from build123d import *

# Parameters (mm, degrees)
SKETCH004_R       = 3.1
PAD001_DEPTH      = 1
PAD001_DEPTH_BACK = 4
SKETCH_R          = 4.1
SKETCH_R_2        = 4
SKETCH_R_3        = 2
PAD_DEPTH         = 12
POCKET_DEPTH      = 70.501
SKETCH002_R       = 3.2
POCKET001_DEPTH   = 1


with BuildPart() as pad001:
    # Sketch004 → Pad001 (new body, two sides)
    with BuildSketch(Plane.XY.offset(5)) as pad001_sk:
        with Locations((0, -29.5)):
            Circle(SKETCH004_R)
    extrude(amount=PAD001_DEPTH)
    extrude(pad001_sk.sketch, amount=-PAD001_DEPTH_BACK)


with BuildPart() as cut:
    # Sketch → Pad (new body)
    with BuildSketch(Plane.XY):
        Polygon((-35.25, 35.05), (-35.25, 19.05), (-5, -35.45), (5, -35.45), (35.25, 19.05), (35.25, 35.05), (23.25, 35.05), (23.25, 23.05), (6, 23.05), (6, 35.05), (-6, 35.05), (-6, 23.05), (-23.25, 23.05), (-23.25, 35.05), align=None)
        with Locations((-29.25, 29.05)):
            Circle(SKETCH_R, mode=Mode.SUBTRACT)
        with Locations((0, 29.05)):
            Circle(SKETCH_R_2, mode=Mode.SUBTRACT)
        with Locations((29.25, 29.05)):
            Circle(SKETCH_R, mode=Mode.SUBTRACT)
        with Locations((-29.25, 19.05)):
            Circle(SKETCH_R_3, mode=Mode.SUBTRACT)
        with Locations((29.25, 19.05)):
            Circle(SKETCH_R_3, mode=Mode.SUBTRACT)
        with Locations((0, -29.45)):
            Circle(SKETCH_R_3, mode=Mode.SUBTRACT)
    extrude(amount=PAD_DEPTH)

    # Sketch001 → Pocket (cut, through all)
    with BuildSketch(Plane(origin=(-35.25, 0, 0), x_dir=(0, -1, 0), z_dir=(-1, 0, 0))):
        Polygon((-19.05, 12), (44.95, 0), (44.95, 12), align=None)
    extrude(amount=-POCKET_DEPTH, mode=Mode.SUBTRACT)

    # Sketch002 → Pocket001 (cut)
    with BuildSketch(Plane.XY.offset(12)):
        with Locations((-29.25, 19.05)):
            Circle(SKETCH002_R)
        with Locations((29.25, 19.05)):
            Circle(SKETCH002_R)
    extrude(amount=-POCKET001_DEPTH, mode=Mode.SUBTRACT)

    # Cut: cut Pad001
    add(pad001.part, mode=Mode.SUBTRACT)


solid = cut.part
Verification items for the finished model (mm, model axes). A direction names the side the tool comes from. Round coordinates to 2 decimals unless told otherwise and drop trailing zeros. Order: outer loops, then holes, each group sorted by start corner. A loop starts at its lowest first (then second) coordinate and runs counter-clockwise, first axis right, second up.
1. Release check for a two-part mould opening along Y. For faces 1 (the flat face through (31, 21, 11)), 2 (the flat face through (15, 23.05, 6)), 3 (the flat face through (-23.25, 29, 6)), 4 (the flat face through (0, -35.45, 1)) record: +Y half, -Y half, draft (parallel to the pull), parting line (faces both ways), or undercut.
Final values:
face 1: undercut
face 2: +Y half
face 3: draft
face 4: -Y half
2. Go/stop test with flat-tipped pins: P1, Ø9.5, axis at x = 29.25, y = 29.05, coming from the +Z side; P2, Ø6, axis at y = -1.5, z = 10.5, coming from the +X side; P3, Ø2, axis at y = -21.5, z = 5.5, coming from the +X side; P4, Ø7, axis at x = 1, y = -28.5, coming from the +Z side. Record where each tip stops, or that it passes through.
Final values:
P1: stops at z = 12
P2: stops at x = 25.12
P3: passes through
P4: stops at z = 3.74
3. Section check A-A on y = 29.05. Record the cut outline in (x, z).
Final values:
outline: (-35.25, 0) - (-33.35, 0) - (-33.35, 12) - (-35.25, 12) - close; (-25.15, 0) - (-23.25, 0) - (-23.25, 12) - (-25.15, 12) - close; (-6, 0) - (-4, 0) - (-4, 12) - (-6, 12) - close; (4, 0) - (6, 0) - (6, 12) - (4, 12) - close; (23.25, 0) - (25.15, 0) - (25.15, 12) - (23.25, 12) - close; (33.35, 0) - (35.25, 0) - (35.25, 12) - (33.35, 12) - close
4. Section check C-C on z = 9.75. Record the cut outline in (x, y).
Final values:
outline: (-35.25, 19.05) - (-28.59, 7.05) - (28.59, 7.05) - (35.25, 19.05) - (35.25, 35.05) - (23.25, 35.05) - (23.25, 23.05) - (6, 23.05) - (6, 35.05) - (-6, 35.05) - (-6, 23.05) - (-23.25, 23.05) - (-23.25, 35.05) - (-35.25, 35.05) - close; hole circle Ø8.2 at (-29.25, 29.05); hole circle Ø4 at (-29.25, 19.05); hole circle Ø8 at (0, 29.05); hole circle Ø8.2 at (29.25, 29.05); hole circle Ø4 at (29.25, 19.05)
5. Section check B-B on x = -29.25. Record the cut outline in (y, z), then the cut area to 3 significant figures.
Final values:
outline: (8.24, 0) - (17.05, 0) - (17.05, 11) - (15.85, 11) - (15.85, 11.4) - (8.24, 9.97) - close; (21.05, 0) - (24.95, 0) - (24.95, 12) - (22.25, 12) - (22.25, 11) - (21.05, 11) - close; (33.15, 0) - (35.05, 0) - (35.05, 12) - (33.15, 12) - close
area: 163 mm2
6. Access from +Z, -Z, +X, -X, +Y, -Y to the whole of each face (thin tool, end or side, straight path). Record for faces 5 (the flat face through (0, 0, 0)), 6 (the flat face through (-6, 29, 6)), 7 (the cylindrical face through (-0.404, -26.426, 2.027)).
Final values:
face 5: -Z, +X, -X, +Y, -Y
face 6: +Z, -Z, +Y
face 7: +Z
7. Thickness scan on L1, parallel to X at y = 19.05, z = 11.7; L2, parallel to Y at x = -29.25, z = 5; L3, parallel to Z at x = -1, y = -32. Record the ranges inside material, lowest first.
Final values:
L1: x = -35.25 to -32.45, -26.05 to 26.05, 32.45 to 35.25
L2: y = 8.24 to 17.05, 21.05 to 24.95, 33.15 to 35.05
L3: z = 0 to 1
8. Section check D-D on x = 0. Record the cut outline in (y, z).
Final values:
outline: (-35.45, 0) - (-31.45, 0) - (-31.45, 1) - (-32.6, 1) - (-32.6, 2.32) - (-35.45, 1.78) - close; (-27.45, 0) - (25.05, 0) - (25.05, 12) - (19.05, 12) - (-26.4, 3.48) - (-26.4, 1) - (-27.45, 1) - close; (33.05, 0) - (35.05, 0) - (35.05, 12) - (33.05, 12) - close
